CAD build for the part. Positions are in the model's coordinates, mm. Coordinates: 2 decimals unless noted, no trailing zeros. Write each loop counter-clockwise with the first axis right and the second up, starting at its lowest first coordinate (ties: lowest second). Pieces come first, ordered by that corner, then holes. Notation, with made-up numbers: (-11, -13) - (18, -13) arc R24 cw to (18, 20) - close; hole circle Ø6 at (63, 10.5). An arc over 180 degrees is marked (long way). Answer in a Markdown table with one row per item. Add a question column.
Q1. Band-saw the part on A-A (x = 0). List the corners of the cut face in (y, z).
Q2. Pin check, flat tips, straight feed: pin 1 (3 mm diameter, centred on x = -5.5, y = 3.5, fed in from -Z); pin 2 (5 mm diameter, centred on y = 8.5, z = 4, fed in from -X); pin 3 (1 mm diameter, centred on x = -6.5, y = 5.5, fed in from +Z); pin 4 (1 mm diameter, centred on y = 4.5, z = -3.5, fed in from +X). Stop position of each tip, or through.
Q3. Two-plate mould, pull along Z, no slides. Class faces 1 (the flat face through (5, 0, 2)), 2 (the flat face through (7.092, 5.427, 4.171)), 3 (the cylindrical face through (-2.4, 5.4, 4.5)): +Z half, -Z half, draft (parallel to the pull), parting line (faces both ways), or undercut.
Q4. Drill centre lines: line 1 along Z through (x, y) = (0, 8.5); line 2 along X through (y, z) = (2.25, -0.75); line 3 along X through (y, z) = (6, -0.5). Where is each one in solid material? Low to high. Write a range as from..to.
Q5. Band-saw the part on B-B (y = 6.25). List the corners of the cut face in (x, z).
```python
from build123d import *

# Parameters (mm, degrees)
EXTRUDE_1_DEPTH     = 11
HOLE_WIZARD_M12_1_D = 10.2


with BuildPart() as part:
    # 草图1 → 凸台-拉伸1 (new body)
    with BuildSketch(Plane(origin=(0, 0, 0), x_dir=(1, 0, 0), z_dir=(0, 1, 0))):
        Polygon((9.5, 0), (4.75, 8.227241336), (-4.75, 8.227241336), (-9.5, 0), (-4.75, -8.227241336), (4.75, -8.227241336), align=None)
    extrude(amount=EXTRUDE_1_DEPTH)

    # M12 螺纹孔1 (through all)
    with Locations(Plane(origin=(0, 11, 0), x_dir=(1, 0, 0), z_dir=(0, 1, 0))):
        with Locations((0, 0)):
            Hole(HOLE_WIZARD_M12_1_D / 2)

    # 草图4 → 切除-旋转1 (revolve, cut)
    with BuildSketch(Plane.XY, mode=Mode.PRIVATE) as cut_revolve_1_sk:
        Polygon((-9.5, 10), (-7.767949192, 11), (-9.5, 11), align=None)
    cut_revolve_1 = revolve(cut_revolve_1_sk.sketch.rotate(Axis((0, 0, 0), (0, 1, 0)), 90), axis=Axis((0, 0, 0), (0, 1, 0)), mode=Mode.SUBTRACT)

    # 镜向1: 切除-旋转1 across plane
    add(cut_revolve_1.mirror(Plane.ZX.offset(5.5)), mode=Mode.SUBTRACT)


solid = part.part
```
Checked values:
| question | item | result |
|---|---|---|
| 1 | outline | (0, -7.77) - (0.27, -8.23) - (10.73, -8.23) - (11, -7.77) - (11, -5.1) - (0, -5.1) - close; (0, 5.1) - (11, 5.1) - (11, 7.77) - (10.73, 8.23) - (0.27, 8.23) - (0, 7.77) - close |
| 2 | pin 1 | stops at z = -8.23 |
| 2 | pin 2 | stops at x = -8.63 |
| 2 | pin 3 | stops at z = 6.06 |
| 2 | pin 4 | stops at x = 7.77 |
| 3 | face 1 | draft |
| 3 | face 2 | +Z half |
| 3 | face 3 | undercut |
| 4 | line 1 | z = -8.23..-5.1, 5.1..8.23 |
| 4 | line 2 | x = -9.07..-5.04, 5.04..9.07 |
| 4 | line 3 | x = -9.21..-5.08, 5.08..9.21 |
| 5 | outline | (-9.5, 0) - (-4.75, -8.23) - (4.75, -8.23) - (9.5, 0) - (4.75, 8.23) - (-4.75, 8.23) - close; hole circle Ø10.2 at (0, 0) |
